from build123d import *

# Parameters (mm, degrees)
F3_DEPTH = 25
F4_SIZE  = 2
F5_R     = 2


with BuildPart() as f1:
    # F0 (on Front) → F1 (revolve)
    with BuildSketch(Plane.XZ):
        Polygon((0, 22), (0, 0), (30, 0), (30, 10), (15, 10), (15, 22), align=None)
    revolve(axis=Axis((0, 0, 11), (0, 0, -1)))

    # F2 (on Top) → F3 (cut)
    with BuildSketch(Plane.XY):
        with BuildLine():
            ThreePointArc((23, -4.25), (26.005204, -3.005204), (27.25, 0))
            ThreePointArc((27.25, 0), (26.005204, 3.005204), (23, 4.25))
            ThreePointArc((23, 4.25), (18.75, 0), (23, -4.25))
        make_face()
        with BuildLine():
            ThreePointArc((23, 4.25), (26.005204, 3.005204), (27.25, 0))
            ThreePointArc((27.25, 0), (26.005204, -3.005204), (23, -4.25))
            Line((23, -4.25), (43, -4.25))
            Line((43, -4.25), (43, 4.25))
            Line((43, 4.25), (23, 4.25))
        make_face()
    extrude(amount=F3_DEPTH, mode=Mode.SUBTRACT)

    # F4
    f4_edges = [f1.edges().sort_by_distance(p)[0] for p in [
        (-30, 0, 0),
        (26.348716, -4.25, 0),
        (18.75, 0, 0),
        (-30, 0, 10),
        (18.75, 0, 10),
    ]]
    chamfer(f4_edges, length=F4_SIZE)

    # F5
    f5_edges = [f1.edges().sort_by_distance(p)[0] for p in [
        (-15, 0, 10),
    ]]
    fillet(f5_edges, radius=F5_R)

    # F0 (on Front) → F6 (revolve)
    with BuildSketch(Plane.XZ):
        Polygon((0, 29.5), (0, 22), (15, 22), (38.5, 22), (38.5, 29.5), (35.5, 29.5), (35.5, 39.5), (30, 39.5), (30, 29.5), align=None)
    revolve(axis=Axis((0, 0, 11), (0, 0, -1)))


solid = f1.part
The model under review builds one solid part; all positions refer to its coordinate system, in mm. A direction names the side the tool comes from. Coordinates: 2 decimals unless noted, no trailing zeros. Write each loop counter-clockwise with the first axis right and the second up, starting at its lowest first coordinate (ties: lowest second). Pieces come first, ordered by that corner, then holes. Notation, with made-up numbers: (77, -23) - (90, -23) arc R10 cw to (90, -12) - close; hole circle Ø5 at (81.5, 53). An arc over 180 degrees is marked (long way). Answer as a JSON object with one key per item and string values. Group by question number.
1. Clearance check with flat-ended pins moving along their axes: pin 1 Ø23 at (x, y) = (-10.5, -7) entering from +Z; pin 2 Ø1.5 at (y, z) = (30, 10) entering from -X; pin 3 Ø12 at (y, z) = (-10.5, 17) entering from -X; pin 4 Ø6 at (y, z) = (-23, 23) entering from +X. State where each tip first meets the part, or that it passes through.
2. Machinability: for faces 1 (the face through (25.65, -5.26, 9.01)), 2 (the face through (18.75, 0.09, 4.96)), 3 (the face through (-28.294, -1.189, 9.681)), 4 (the face through (-7.696, 34.656, 34.57)), which of the approach directions +Z, -Z, +X, -X, +Y, -Y give a long, thin tool a straight path to every point of the face, cutting with its end or side? Answer none if there is none.
3. To check wall thickness, follow probe 1 along X at (y, z) = (0, 34.75); probe 2 along Z at (x, y) = (-1.5, 12). State the ranges of each line that lie inside material, in increasing order.
4. Mouldability with a two-part tool opening along X and no side actions: class faces 5 (the face through (1, 17, 22)), 6 (the face through (-28.1, -1.181, 0.125)), 7 (the face through (-29.97, -1.32, 34.43)) as pulls with the +X half, pulls with the -X half, needs draft (parallel to the pull), parting line crosses it, or undercut.
5. Add section B-B (y = 32). Give the boundary of the cut face in (x, z).
6. Add section D-D (z = 4). Give the boundary of the cut face in (x, y), plus the area to 3 significant figures.
7. Add section A-A (x = 0). Give the boundary of the cut face in (y, z), plus the area to 3 significant figures.
8. Add section C-C (z = 33.5). Give the boundary of the cut face in (x, y), plus the area to 3 significant figures.
Findings:
{
 "1": {"pin 1": "z = 29.5", "pin 2": "through", "pin 3": "x = -37.82", "pin 4": "x = 32.9"},
 "2": {"face 1": "+X", "face 2": "-Z, +X", "face 3": "none", "face 4": "+Z"},
 "3": {"probe 1": "-35.5 to -30, 30 to 35.5", "probe 2": "0 to 29.5"},
 "4": {"face 5": "needs draft", "face 6": "parting line crosses it", "face 7": "undercut"},
 "5": {"outline": "(-21.41, 22) - (21.41, 22) - (21.41, 29.5) - (15.37, 29.5) - (15.37, 39.5) - (-15.37, 39.5) - (-15.37, 29.5) - (-21.41, 29.5) - close"},
 "6": {"outline": "(23, -4.25) arc R4.25 cw to (23, 4.25) - (29.7, 4.25) arc R30 ccw (long way) to (29.7, -4.25) - close", "area": "2,740 mm²"},
 "7": {"outline": "(-38.5, 22) - (-15, 22) - (-15, 12) arc R2 cw to (-17, 10) - (-28, 10) - (-30, 8) - (-30, 2) - (-28, 0) - (28, 0) - (30, 2) - (30, 8) - (28, 10) - (17, 10) arc R2 cw to (15, 12) - (15, 22) - (38.5, 22) - (38.5, 29.5) - (35.5, 29.5) - (35.5, 39.5) - (30, 39.5) - (30, 29.5) - (-30, 29.5) - (-30, 39.5) - (-35.5, 39.5) - (-35.5, 29.5) - (-38.5, 29.5) - close", "area": "1,640 mm²"},
 "8": {"outline": "circle Ø71 at (0, 0); hole circle Ø60 at (0, 0)", "area": "1,130 mm²"}
}
